Input: dimensioned drawing with shaded views. Units: mm. Origin: part minimum x, y, z. A direction names the side the tool comes from. Give positions to 0.01 mm unless a question says otherwise; leave off trailing zeros. Write each loop counter-clockwise with the first axis right and the second up, starting at its lowest first coordinate (ties: lowest second). Pieces come first, ordered by that corner, then holes. Notation, with made-up numbers: (8, -21.5) -> (20, -21.5) arc R37 ccw to (20, 16.5) -> close; hole circle Ø5 at (-17, -36.75). An arc over 180 degrees is marked (long way). Answer as a JSON object with one key per item and string values. Group by question number.
(1) Section query C-C on y = 32. Output: boundary loops of the cut face in (x, z), plus the area to 3 significant figures.
(2) Material intervals for probe 1 along X at (y, z) = (26.5, 6.75); probe 2 along X at (y, z) = (31, 1.5); probe 3 along X at (y, z) = (46, 6.75), sorted ascending.
(3) Contact query for flat-ended pins moving along their axis: pin 1 Ø3 at (y, z) = (33.5, 5.5) entering from -X; pin 2 Ø1 at (y, z) = (77, 8) entering from +X; pin 3 Ø1.5 at (y, z) = (40.5, 1.5) entering from +X. Output: stop coordinate, or through.
(4) Draft query along X for the marked faces 3, 4, 5 and 6. Return one class per face: +X half, -X half, draft (parallel to the pull), parting line (faces both ways), or undercut.
(5) Section query B-B on z = 2.5. Output: boundary loops of the cut face in (x, y), plus the area to 4 significant figures.
(6) Set-up query: the marked faces 1 and 2. Return all of +Z, -Z, +X, -X, +Y, -Y with unobstructed straight access to the full face (end or side cutting, diameter ignored); none if empty.
(7) Section query A-A on x = 52. Output: boundary loops of the cut face in (y, z).
(8) Section query D-D on y = 61. Output: boundary loops of the cut face in (x, z).
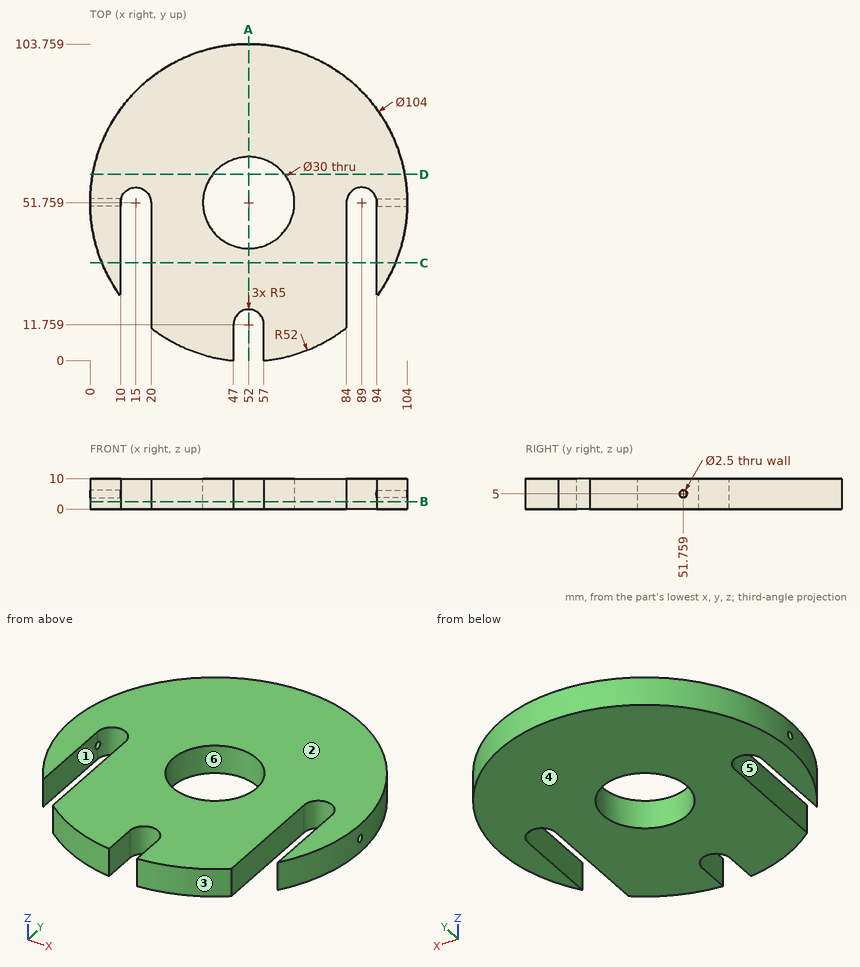
Answer list:
{
 "1": {"outline": "(3.9, 0) -> (10, 0) -> (10, 10) -> (3.9, 10) -> close; (20, 0) -> (84, 0) -> (84, 10) -> (20, 10) -> close; (94, 0) -> (100.1, 0) -> (100.1, 10) -> (94, 10) -> close", "area": "762 mm2"},
 "2": {"probe 1": "6.55 to 10, 20 to 84, 94 to 97.45", "probe 2": "4.32 to 10, 20 to 84, 94 to 99.68", "probe 3": "0.32 to 10, 20 to 38.15, 65.85 to 84, 94 to 103.68"},
 "3": {"pin 1": "x = 2.77", "pin 2": "x = 97.74", "pin 3": "x = 102.93"},
 "4": {"face 3": "+X half", "face 4": "draft", "face 5": "undercut", "face 6": "undercut"},
 "5": {"outline": "(10, 21.1) -> (10, 51.76) arc R5 cw to (20, 51.76) -> (20, 10.77) arc R52 ccw to (47, 0) -> (47, 11.76) arc R5 cw to (57, 11.76) -> (57, 0) arc R52 ccw to (84, 10.77) -> (84, 51.76) arc R5 cw to (94, 51.76) -> (94, 21.1) arc R52 ccw (long way) to start; hole circle Ø30 at (52, 51.76)", "area": "6,825 mm2"},
 "6": {"face 1": "+Z, -Z, -Y", "face 2": "+Z, +X, -X, +Y, -Y"},
 "7": {"outline": "(16.76, 0) -> (36.76, 0) -> (36.76, 10) -> (16.76, 10) -> close; (66.76, 0) -> (103.76, 0) -> (103.76, 10) -> (66.76, 10) -> close"},
 "8": {"outline": "(0.83, 0) -> (40.18, 0) -> (40.18, 10) -> (0.83, 10) -> close; (63.82, 0) -> (103.17, 0) -> (103.17, 10) -> (63.82, 10) -> close"}
}
